Design review of the part shown in the three views and the two pictorial views. Dimensions are in mm from the part's minimum x, y and z. Coordinates: 2 decimals unless noted, no trailing zeros. Write each loop counter-clockwise with the first axis right and the second up, starting at its lowest first coordinate (ties: lowest second). Pieces come first, ordered by that corner, then holes. Notation, with made-up numbers: (41.5, -8.5) -> (77.5, -8.5) arc R31 ccw to (77.5, 23.5) -> close; hole circle Ø11 at (63, 20.5). An arc over 180 degrees is marked (long way). Answer in a Markdown table with one row per item. Add a question column.
Item 1: Take a section at B-B, the plane x = 11.5. Write out the cut boundary in (y, z).
Item 2: Draft analysis for pull direction Y (two halves, no side actions). For the marked faces 1, 2 and 3, state which applies: released by +Y, released by -Y, zero draft, split by the parting line, or undercut.
Item 3: Clearance check with flat-ended pins moving along their axes: P1, Ø5, axis at x = 19.26, y = 10.72, coming from the +Z side; P2, Ø1, axis at y = 37.5, z = 1, coming from the -X side (1 decimal); P3, Ø3, axis at x = 29.16, y = 20.62, coming from the +Z side; P4, Ø1, axis at y = 22, z = 3, coming from the -X side (1 decimal). State where each tip first meets the part, or that it passes through.
Item 4: To check wall thickness, follow line 1 (Y direction, x = 30, z = 1.45) (1 decimal); line 2 (X direction, y = 10, z = 1.3) (1 decimal); line 3 (Y direction, x = 28.5, z = 0.35) (1 decimal). State the ranges of each line that lie inside material, in increasing order.
Item 5: Take a section at C-C, the plane z = 1.05. Write out the cut boundary in (x, y) (1 decimal).
Item 6: Take a section at A-A, the plane y = 26.5. Write out the cut boundary in (x, z).
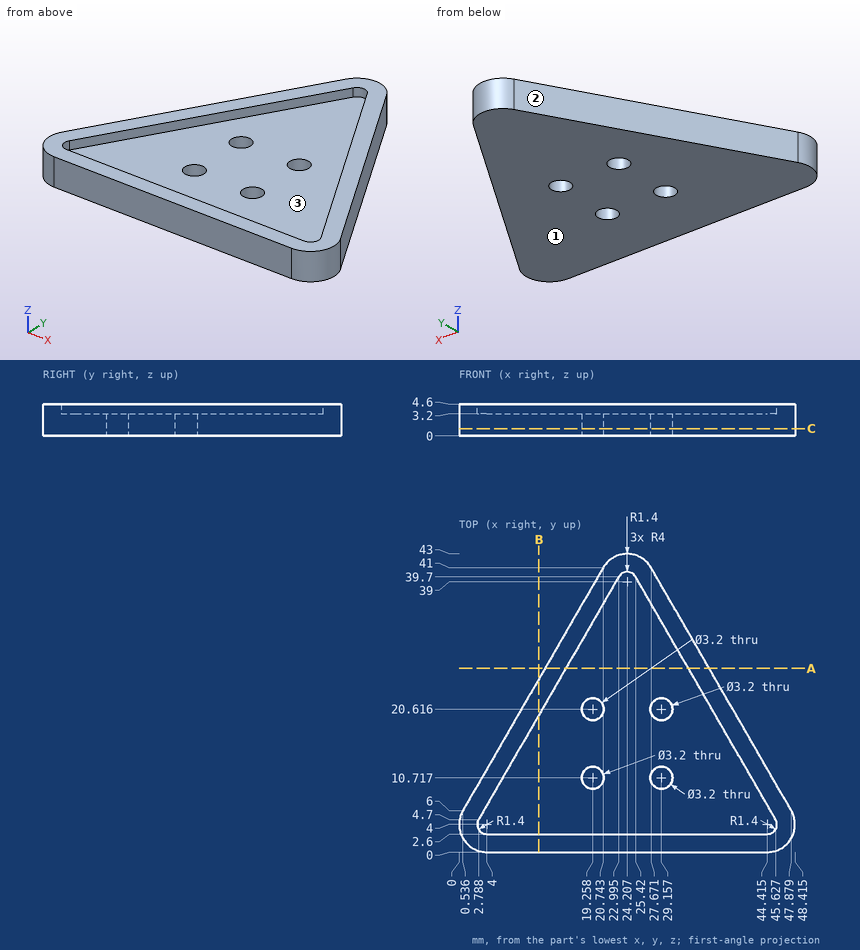
Answers:
| question | item | result |
|---|---|---|
| 1 | outline | (0, 0) -> (24.99, 0) -> (24.99, 4.6) -> (19.79, 4.6) -> (19.79, 3.2) -> (2.6, 3.2) -> (2.6, 4.6) -> (0, 4.6) -> close |
| 2 | face 1 | zero draft |
| 2 | face 2 | released by +Y |
| 2 | face 3 | undercut |
| 3 | P1 | stops at z = 3.2 |
| 3 | P2 | stops at x = 18.4 |
| 3 | P3 | passes through |
| 3 | P4 | stops at x = 9.5 |
| 4 | line 1 | y = 0 to 9.4, 12.1 to 19.3, 22 to 37 |
| 4 | line 2 | x = 2.8 to 17.8, 20.7 to 27.7, 30.6 to 45.6 |
| 4 | line 3 | y = 0 to 9.3, 12.2 to 19.2, 22.1 to 39.6 |
| 5 | outline | (0.5, 6) arc R4 ccw to (4, 0) -> (44.4, 0) arc R4 ccw to (47.9, 6) -> (27.7, 41) arc R4 ccw to (20.7, 41) -> close; hole circle Ø3.2 at (19.3, 10.7); hole circle Ø3.2 at (19.3, 20.6); hole circle Ø3.2 at (29.2, 10.7); hole circle Ø3.2 at (29.2, 20.6) |
| 6 | outline | (12.37, 0) -> (36.04, 0) -> (36.04, 4.6) -> (33.04, 4.6) -> (33.04, 3.2) -> (15.37, 3.2) -> (15.37, 4.6) -> (12.37, 4.6) -> close |
